Here's the drawing with two shaded views (mm, measured from the low corner). I have some questions. Give positions to 0.01 mm unless a question says otherwise; leave off trailing zeros. Write each loop counter-clockwise with the first axis right and the second up, starting at its lowest first coordinate (ties: lowest second). Pieces come first, ordered by that corner, then holes. Notation, with made-up numbers: (38.25, -7) - (67.25, -7) arc R11 cw to (67.25, 3) - close; hole circle Ø2 at (-5.5, 47.5). An arc over 180 degrees is marked (long way). Use one line per item in the form item = value.
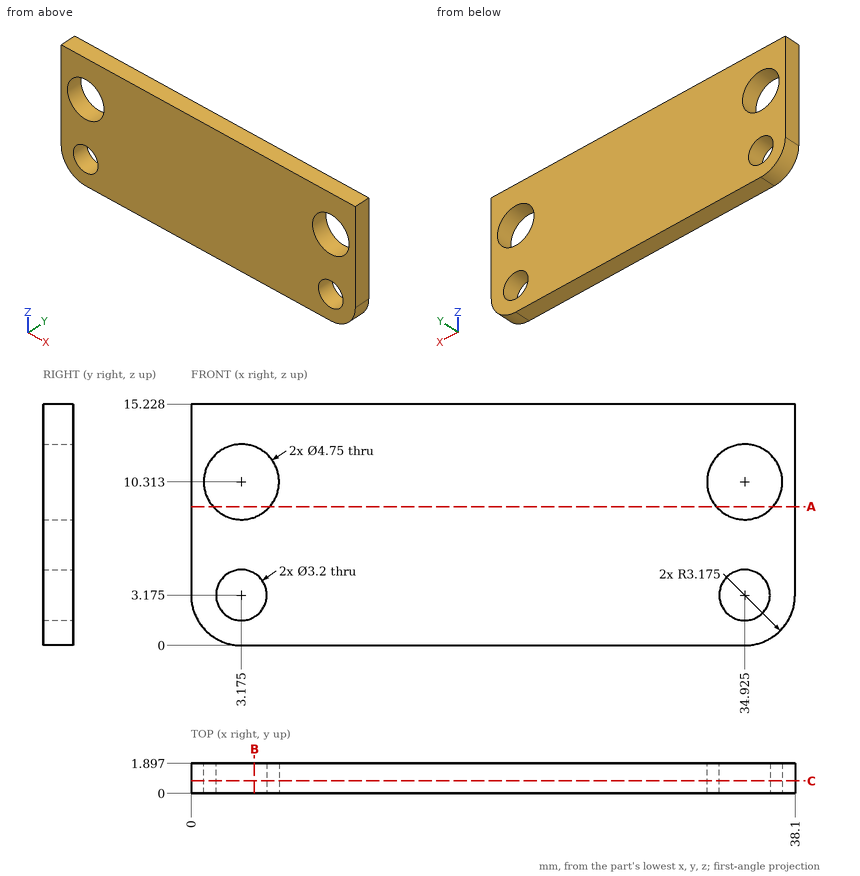
1. If I drill on line 1 (X direction, y = 1.65, z = 10); line 2 (Z direction, x = 4, y = 1.8) (1 decimal); line 3 (X direction, y = 1.05, z = 8.5), over which ranges is the centre line in solid material (lowest first)? Write a range as from..to.
Response values:
line_1 = 0..0.82, 5.53..32.57, 37.28..38.1
line_2 = 0..1.8, 4.5..8.1, 12.5..15.2
line_3 = 0..1.64, 4.71..33.39, 36.46..38.1
2. Imagine slicing it at B-B, the plane x = 4. List the corners of the cut face in (y, z) for me (1 decimal).
Response values:
outline = (0, 0) - (1.9, 0) - (1.9, 1.8) - (0, 1.8) - close; (0, 4.5) - (1.9, 4.5) - (1.9, 8.1) - (0, 8.1) - close; (0, 12.5) - (1.9, 12.5) - (1.9, 15.2) - (0, 15.2) - close
3. Imagine slicing it at C-C, the plane y = 0.8. State how many separate pieces and enclosed holes the cut face has, and give its area (3 significant figures).
Response values:
separate_pieces = 1
enclosed_holes = 4
area = 524 mm²
4. Imagine slicing it at A-A, the plane z = 8.75. List the corners of the cut face in (x, y) for me.
Response values:
outline = (0, 0) - (1.39, 0) - (1.39, 1.9) - (0, 1.9) - close; (4.96, 0) - (33.14, 0) - (33.14, 1.9) - (4.96, 1.9) - close; (36.71, 0) - (38.1, 0) - (38.1, 1.9) - (36.71, 1.9) - close
